```python
from build123d import *

# Parameters (mm, degrees)
BOSS_EXTRUDE5_DEPTH      = 26
BOSS_EXTRUDE5_DEPTH_BACK = 26
RIB1_REACH               = 62.682
SKETCH8_WALL_W           = 164.057376466
SKETCH8_WALL_H           = 8


with BuildPart() as part:
    # Sketch7 → Boss-Extrude5 (new, two sides: drawn at the far end of the back side and taken through both)
    with BuildSketch(Plane.XY.offset(-BOSS_EXTRUDE5_DEPTH_BACK)):
        with BuildLine():
            Line((-17.60590988, 40), (-8.880775936, 40))
            ThreePointArc((-8.880775936, 40), (0, 31.119224064), (8.880775936, 40))
            Line((8.880775936, 40), (17.60590988, 40))
            ThreePointArc((17.60590988, 40), (13.949814643, 29.258923046), (4.5, 22.978893611))
            Line((4.5, 22.978893611), (4.5, 4.5))
            Line((4.5, 4.5), (37.5, 4.5))
            Line((37.5, 4.5), (37.5, -4.5))
            Line((37.5, -4.5), (-37.5, -4.5))
            Line((-37.5, -4.5), (-37.5, 4.5))
            Line((-37.5, 4.5), (-4.5, 4.5))
            Line((-4.5, 4.5), (-4.5, 22.978893611))
            ThreePointArc((-4.5, 22.978893611), (-13.949814643, 29.258923046), (-17.60590988, 40))
        make_face()
    extrude(amount=BOSS_EXTRUDE5_DEPTH + BOSS_EXTRUDE5_DEPTH_BACK)

    # Sketch8 wall → Rib1 (add, up to next)
    with BuildSketch(Plane(origin=(27.55295494, 22.25, 0), x_dir=(0.488866930082, -0.872358369406, 0), z_dir=(0.872358369406, 0.488866930082, 0)), mode=Mode.PRIVATE) as rib1_sk1:
        Rectangle(SKETCH8_WALL_W, SKETCH8_WALL_H)
    rib1_tool1 = extrude(rib1_sk1.sketch, amount=-RIB1_REACH, mode=Mode.PRIVATE) - part.part
    add(rib1_tool1.solids().sort_by_distance((27.55295494, 22.25, 0))[0])


solid = part.part
```
For this review, take the finished solid that the model builds, in its own axes (mm). A direction names the side the tool comes from. Round coordinates to 2 decimals unless told otherwise and drop trailing zeros. Order: outer loops, then holes, each group sorted by start corner. A loop starts at its lowest first (then second) coordinate and runs counter-clockwise, first axis right, second up.
Q1. We need section D-D, the plane x = -31. Give the boundary of the cut face in (y, z), plus the area to 3 significant figures.
Findings below:
outline: (-4.5, -26) - (4.5, -26) - (4.5, 26) - (-4.5, 26) - close
area: 468 mm2
Q2. We need section C-C, the plane x = 0. Give the boundary of the cut face in (y, z), plus the area to 3 significant figures.
Findings below:
outline: (-4.5, -26) - (31.12, -26) - (31.12, 26) - (-4.5, 26) - close
area: 1,850 mm2
Q3. We need section B-B, the plane x = -16. Give the boundary of the cut face in (y, z).
Findings below:
outline: (-4.5, -26) - (4.5, -26) - (4.5, 26) - (-4.5, 26) - close; (32.65, -26) - (40, -26) - (40, 26) - (32.65, 26) - close
Q4. Wall thickness on line 1 (X direction, y = 18.5, z = -19); line 2 (Y direction, x = -0.5, z = -15.5): over which ranges is each line inside the solid? List them lowest first.
Findings below:
line 1: x = -4.5 to 4.5
line 2: y = -4.5 to 31.13
Q5. Machinability: for faces 5 (the flat face through (1, 13, -26)), 6 (the flat face through (18, 17, -4)), 7 (the flat face through (37.5, 0, 0)), 8 (the flat face through (21, 4.5, 15)), 9 (the flat face through (-4.5, 14, 0)), which of the approach directions +Z, -Z, +X, -X, +Y, -Y give a long, thin tool a straight path to every point of the face, cutting with its end or side? Answer none if there is none.
Findings below:
face 5: -Z, +X, -X, +Y, -Y
face 6: -Z, +X
face 7: +Z, -Z, +X, +Y, -Y
face 8: +Z, +X
face 9: +Z, -Z, -X
Q6. Insertion check: P1, Ø1.5, axis at y = 15, z = -6.5, coming from the +X side; P2, Ø6, axis at x = -29, z = -19, coming from the +Y side. Each pin has a flat end and moves straight along its axis. Give the tip position at first contact, or say it passes through.
Findings below:
P1: stops at x = 4.5
P2: stops at y = 4.5
Q7. We need section A-A, the plane z = 17.5. Give the boundary of the cut face in (x, y).
Findings below:
outline: (-37.5, -4.5) - (37.5, -4.5) - (37.5, 4.5) - (4.5, 4.5) - (4.5, 22.98) arc R17.61 ccw to (17.61, 40) - (8.88, 40) arc R8.88 cw to (-8.88, 40) - (-17.61, 40) arc R17.61 ccw to (-4.5, 22.98) - (-4.5, 4.5) - (-37.5, 4.5) - close
Q8. Mouldability with a two-part tool opening along Y and no side actions: class faces 1 (the flat face through (-13, 40, 0)), 2 (the flat face through (1, -4.5, 0)), 3 (the cylindrical face through (14.05, 29.39, -15.15)), 4 (the flat face through (-37.5, 0, 0)) as pulls with the +Y half, pulls with the -Y half, needs draft (parallel to the pull), parting line crosses it, or undercut.
Findings below:
face 1: pulls with the +Y half
face 2: pulls with the -Y half
face 3: undercut
face 4: needs draft
